Autodesk Inventor part; units mm, degrees
ref_plane "YZ Plane" through (0, 0, 0) normal (1, 0, 0) x (0, 1, 0)
ref_plane "XZ Plane" through (0, 0, 0) normal (0, 1, 0) x (-1, 0, 0)
ref_plane "XY Plane" through (0, 0, 0) normal (0, 0, 1) x (1, 0, 0)
sketch "Sketch1" plane through (0, 0, 0) normal (0, 1, 0) x (-1, 0, 0)
  line L0 (22, 20) -> (-22, 20)
  line L1 (-22, 20) -> (-22, -20)
  line L2 (-22, -20) -> (22, -20)
  line L3 (22, -20) -> (22, 20)
  line L4 (22, 20) -> (-22, -20) construction
  line L5 (-22, 20) -> (22, -20) construction
  point P0 (0, 0)
  dimension "CUBE_DIM" = 40
  dimension "d1" = 44
extrude "Extrusion1" add sketch "Sketch1" along normal blind 5.4
sketch "Sketch2" plane through (0, 5.4, 0) normal (0, 1, 0) x (1, 0, 0)
  line L0 (-22, -31) -> (22, -31)
  line L1 (22, -31) -> (22, 31)
  line L2 (22, 31) -> (-22, 31)
  line L3 (-22, 31) -> (-22, -31)
  line L4 (-22, -31) -> (22, 31) construction
  line L5 (22, -31) -> (-22, 31) construction
  line L6 (-22, 20) -> (-22, -20)
  line L7 (-22, -20) -> (22, -20)
  line L8 (22, 20) -> (-22, 20)
  line L9 (-22, 20) -> (22, 20)
  point P0 (0, 0)
  dimension "BASE_LENGTH" = 62
  dimension "BASE_WIDTH" = 44
extrude "Extrusion2" add sketch "Sketch2" against normal blind 5.4
sketch "Sketch5" plane through (0, 0, 0) normal (0, -1, 0) x (1, 0, 0)
  line L0 (22, 20) -> (20, 20)
  line L1 (20, 20) -> (20, -20)
  line L2 (20, -20) -> (22, -20)
  line L3 (22, -20) -> (22, 20)
  line L4 (22, 31) -> (22, -31)
  point P0 (0, 0)
  dimension "d31" = 40
  dimension "d32" = 20
  dimension "d33" = 0
  dimension "d34" = 2
extrude "Extrusion3" add sketch "Sketch5" along normal blind 2
sketch "Sketch3" plane through (0, 5.4, 0) normal (0, 1, 0) x (1, 0, 0)
  circle A0 centre (0, 0) radius 2.9522
  line L0 (20, 20) -> (20, -20)
  dimension "d35" = 20
hole "Hole1" at (0, 5.4, 0) direction (0, -1, 0) diameter 3.242 depth 5.4 counterbore diameter 4 counterbore depth 1.9
sketch "Sketch4" plane through (0, 0, 0) normal (0, -1, 0) x (1, 0, 0)
  circle A0 centre (0, -25) radius 1.0924
  circle A1 centre (0, 25) radius 1.3036
  line L0 (-22, -31) -> (22, -31)
  line L1 (22, 31) -> (-22, 31)
  point P0 (0, 0)
  point P1 (-22, -29)
  point P2 (-22, 29)
  point P3 (22, -31)
  point P4 (-22, 31)
  dimension "d22" = 6
  dimension "d23" = 6
hole "Hole2" at (0, 0, 25) at (0, 0, -25) direction (0, 1, 0) diameter 4.31 depth 12.3 counterbore diameter 7.94 counterbore depth 2.4
equation "\"PLATFORM_HEIGHT\" = BEAM_HEIGHT - 0.5 * CUBE_DIM"
equation "\"BASE_LENGTH\" = CUBE_DIM + 2 * WING_SIZE"
equation "\"d13\" = PLATFORM_HEIGHT"
equation "\"WING_SIZE\" = 11"
equation "\"BEAM_HEIGHT\" = 25.4"
properties part number "EOM mount"
Geometry: final body of the model. Coordinates: model frame, mm. A direction names the side the tool comes from. Give positions to 0.01 mm unless a question says otherwise; leave off trailing zeros. Loops run counter-clockwise (first coordinate to the right, second up) from the corner with the lowest first, then second, coordinate; pieces in that order, holes last. Notation, with made-up numbers: (59, 43) -> (69, 43) arc R15 cw to (69, 64) -> close; hole circle Ø8 at (60.5, 17). An arc over 180 degrees is marked (long way). Return JSON: item names as keys, results as strings.
Item 1: Section A-A, the plane z = -25. Output: boundary loops of the cut face in (x, y) (3 decimals), plus the area to 3 significant figures.
Filled in:
{"outline": "(-22, 0) -> (-3.97, 0) -> (-3.97, 2.4) -> (-2.155, 2.4) -> (-2.155, 5.4) -> (-22, 5.4) -> close; (2.155, 2.4) -> (3.97, 2.4) -> (3.97, 0) -> (22, 0) -> (22, 5.4) -> (2.155, 5.4) -> close", "area": "206 mm^2"}
Item 2: Line query: line 1 (Z direction, x = 0, y = 1.05); line 2 (Z direction, x = 0, y = 3.85) (3 decimals); line 3 (X direction, y = 3, z = -25) (3 decimals). Output: solid intervals per line, ascending.
Filled in:
{"line 1": "-31 to -28.97, -21.03 to -1.62, 1.62 to 21.03, 28.97 to 31", "line 2": "-31 to -27.155, -22.845 to -2, 2 to 22.845, 27.155 to 31", "line 3": "-22 to -2.155, 2.155 to 22"}
Item 3: Section C-C, the plane z = -17. Output: boundary loops of the cut face in (x, y), plus the area to 3 significant figures.
Filled in:
{"outline": "(-22, 0) -> (20, 0) -> (20, -2) -> (22, -2) -> (22, 5.4) -> (-22, 5.4) -> close", "area": "242 mm^2"}
Item 4: Pin query (flat end, axial travel): P1, Ø3, axis at x = 0, z = 0, coming from the +Y side; P2, Ø4, axis at x = 1, z = -23.5, coming from the -Y side; P3, Ø6.5, axis at x = 0.5, z = 24, coming from the -Y side; P4, Ø0.6, axis at x = 21.5, y = -1, coming from the +Z side. Return the tip coordinate at first contact, or that it passes through.
Filled in:
{"P1": "through", "P2": "y = 2.4", "P3": "y = 0", "P4": "z = 20"}
Item 5: Section D-D, the plane x = -15.5. Output: boundary loops of the cut face in (y, z), plus the area to 3 significant figures.
Filled in:
{"outline": "(0, -31) -> (5.4, -31) -> (5.4, 31) -> (0, 31) -> close", "area": "335 mm^2"}
Item 6: Mould query, pull axis Z, two halves, no side actions, for faces 4 (the flat face through (-22, 3, 0)), 5 (the flat face through (2, 2.4, 23)), 6 (the flat face through (0, 3, -31)). Classes: released by +Z, released by -Z, zero draft, split by the parting line, or undercut.
Filled in:
{"face 4": "zero draft", "face 5": "undercut", "face 6": "released by -Z"}
Item 7: Section B-B, the plane x = 0. Output: boundary loops of the cut face in (y, z) (3 decimals), plus the area to 3 significant figures.
Filled in:
{"outline": "(0, -31) -> (5.4, -31) -> (5.4, -27.155) -> (2.4, -27.155) -> (2.4, -28.97) -> (0, -28.97) -> close; (0, -21.03) -> (2.4, -21.03) -> (2.4, -22.845) -> (5.4, -22.845) -> (5.4, -2) -> (3.5, -2) -> (3.5, -1.621) -> (0, -1.621) -> close; (0, 1.621) -> (3.5, 1.621) -> (3.5, 2) -> (5.4, 2) -> (5.4, 22.845) -> (2.4, 22.845) -> (2.4, 21.03) -> (0, 21.03) -> close; (0, 28.97) -> (2.4, 28.97) -> (2.4, 27.155) -> (5.4, 27.155) -> (5.4, 31) -> (0, 31) -> close", "area": "252 mm^2"}
Item 8: Access query for faces 1 (the flat face through (21, -1, -20)), 2 (the flat face through (2, 2.4, -27)), 3 (the flat face through (21, -1, 20)). Directions: +Z, -Z, +X, -X, +Y, -Y. A direction counts if a zero-diameter tool reaches every point of the face in a straight line with its end or side. Return the directions, or none.
Filled in:
{"face 1": "-Z, +X, -X, -Y", "face 2": "-Y", "face 3": "+Z, +X, -X, -Y"}
